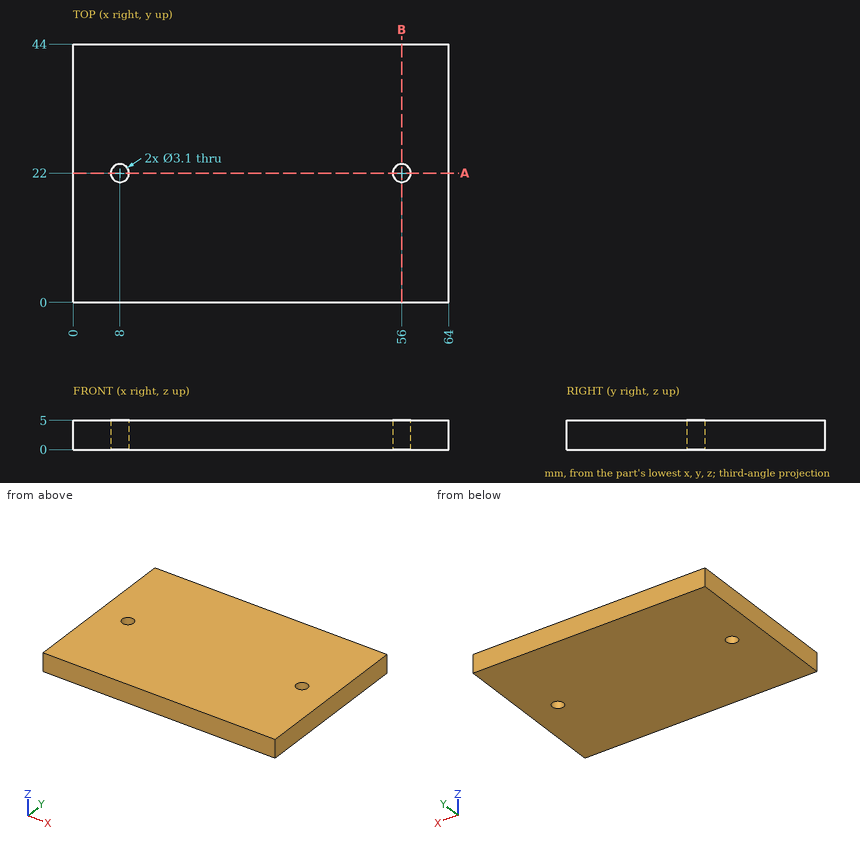
Geometry check sheet. Reference: drawing and pictorial views, mm from the part's lowest x, y, z. Round coordinates to 2 decimals unless told otherwise and drop trailing zeros. Order: outer loops, then holes, each group sorted by start corner. A loop starts at its lowest first (then second) coordinate and runs counter-clockwise, first axis right, second up. Notation, with made-up numbers: (1.25, 9) - (24.25, 9) arc R32 cw to (24.25, 36) - close; hole circle Ø6 at (25.25, 41.25). An arc over 180 degrees is marked (long way). Write item = value, one per line.
Q1. Thickness scan on line 1 along X through (y, z) = (23, 2); line 2 along Y through (x, z) = (56, 3.25); line 3 along Y through (x, z) = (57, 1.55). Record the ranges inside material, lowest first.
Computed:
line_1 = 0 to 6.82, 9.18 to 54.82, 57.18 to 64
line_2 = 0 to 20.45, 23.55 to 44
line_3 = 0 to 20.82, 23.18 to 44
Q2. Section check B-B (x = 56). Record the boundary of the cut face in (y, z), and give its area (4 significant figures).
Computed:
outline = (0, 0) - (20.45, 0) - (20.45, 5) - (0, 5) - close; (23.55, 0) - (44, 0) - (44, 5) - (23.55, 5) - close
area = 204.5 mm^2
Q3. Section check A-A (y = 22). Record the boundary of the cut face in (x, z).
Computed:
outline = (0, 0) - (6.45, 0) - (6.45, 5) - (0, 5) - close; (9.55, 0) - (54.45, 0) - (54.45, 5) - (9.55, 5) - close; (57.55, 0) - (64, 0) - (64, 5) - (57.55, 5) - close
